Read the model definition and answer for the solid it produces. Units are mm, in the model's axes. A direction names the side the tool comes from. Coordinates: 2 decimals unless noted, no trailing zeros. Loops run counter-clockwise (first coordinate to the right, second up) from the corner with the lowest first, then second, coordinate; pieces in that order, holes last. Notation, with made-up numbers: (14, 46) - (65, 46) arc R19 cw to (65, 57) - close; hole circle Ø8 at (81.5, 8). An arc over 180 degrees is marked (long way). Use CSV: the item, a comma, the result in double quotes.
Autodesk Inventor part; units mm, degrees
ref_plane "Start Plane" through (0, 0, 0) normal (1, 0, 0) x (0, 1, 0)
ref_plane "XZ Plane" through (0, 0, 0) normal (0, 1, 0) x (-1, 0, 0)
ref_plane "XY Plane" through (0, 0, 0) normal (0, 0, 1) x (1, 0, 0)
sketch "Main Sketch" plane through (0, 0, 0) normal (0, 0, 1) x (1, 0, 0)
  line L0 (0, 0) -> (77, 0)
  line L1 (0, 0) -> (0, 16.5)
  line L2 (42, 16.5) -> (42, 15)
  line L3 (0, 16.5) -> (42, 16.5)
  line L4 (77, 15) -> (77, 0)
  line L5 (42, 15) -> (77, 15)
  dimension "d3" = 33
  dimension "d4" = 30
revolve "Revolution1" add sketch "Main Sketch" angle 360 about axis through (0, 0, 0) along (1, 0, 0)
chamfer "Chamfer1" distance 0.5 angle 45 1 edges at (0, -16.5, 0) measured on face at (28, 16.4465, -1.3277)
fillet "Fillet1" radius 5 1 edges at (42, -16.5, 0)
equation "\"Length\" = 77"
properties part number "Shaft" material "Steel"
Q1. A tool of negligible diameter and unlimited length cuts with its end or side. For faces 1 (the face through (59.745, -14.985, 0.66)), 2 (the face through (77, 0, 0)), from which of +Z, -Z, +X, -X, +Y, -Y can it reach the whole face along a straight path? Write none if from no direction.
Reported:
face 1,"+X"
face 2,"+Z, -Z, +X, +Y, -Y"
Q2. The part is cut by section C-C on x = 8. Determine the outline of the cut face in (y, z).
Reported:
outline,"circle Ø33 at (0, 0)"
Q3. The part is cut by section D-D on x = 68. Determine the outline of the cut face in (y, z).
Reported:
outline,"circle Ø30 at (0, 0)"
Q4. The part is cut by section A-A on y = 0. Determine the outline of the cut face in (x, z).
Reported:
outline,"(0, -16) - (0.5, -16.5) - (38.43, -16.5) arc R5 ccw to (42, -15) - (77, -15) - (77, 15) - (42, 15) arc R5 ccw to (38.43, 16.5) - (0.5, 16.5) - (0, 16) - close"
Q5. Find the intervals of material crossed by probe 1 along Z at (x, y) = (49.5, 0.5); probe 2 along Z at (x, y) = (63.5, 3); probe 3 along Y at (x, z) = (70, -4.5), in increasing order. Write a range as [from, to].
Reported:
probe 1,"z = [-14.99, 14.99]"
probe 2,"z = [-14.7, 14.7]"
probe 3,"y = [-14.31, 14.31]"
Q6. Given P1, Ø3, axis at x = 30.5, z = -8, coming from the +Y side; P2, Ø1, axis at x = 45, y = -3.5, coming from the -Z side; P3, Ø6, axis at x = 35, z = -3.5, coming from the +Y side, each flat-ended and moving along its own axis, determine where each tip first touches the part or whether it passes through.
Reported:
P1,"stops at y = 15.17"
P2,"stops at z = -14.7"
P3,"stops at y = 16.49"
